Design review of the part built by this model. Coordinates are the model's own, in mm. A direction names the side the tool comes from. Coordinates: 2 decimals unless noted, no trailing zeros. Write each loop counter-clockwise with the first axis right and the second up, starting at its lowest first coordinate (ties: lowest second). Pieces come first, ordered by that corner, then holes. Notation, with made-up numbers: M -0.5,32 L 22.5,32 A13 ccw 22.5,39 Z; hole C 79.25,7 d7. An arc over 180 degrees is marked long. Return JSON: item names as keys, results as strings. Group by question number.
```python
from build123d import *

# Parameters (mm, degrees)
SKETCH1_W           = 34.124427795
SKETCH1_H           = 26.117733668
SKETCH1_R           = 1.70000044
BOSS_EXTRUDE3_DEPTH = 2.5


with BuildPart() as part:
    # Sketch1 → Boss-Extrude3 (new body)
    with BuildSketch(Plane.XY):
        with Locations((17.062213898, 13.058866834)):
            Rectangle(SKETCH1_W, SKETCH1_H)
        with Locations((17.170001507, 3.630000591)):
            Circle(SKETCH1_R, mode=Mode.SUBTRACT)
        with Locations((17.170000399, 22.630012776)):
            Circle(SKETCH1_R, mode=Mode.SUBTRACT)
        Polygon((30.684032724, 15.567255888), (28.662081374, 15.567255888), (28.662081374, 19.434703738), (5.372492357, 19.434703738), (5.372492357, 6.850018518), (28.662081374, 6.850018518), (28.662081374, 10.717466368), (30.684032724, 10.717466368), align=None, mode=Mode.SUBTRACT)
    extrude(amount=BOSS_EXTRUDE3_DEPTH)


solid = part.part
```
Item 1: Machinability: for faces 1 (the flat face through (21, 5, 0)), 2 (the flat face through (5.372, 13, 1)), which of the approach directions +Z, -Z, +X, -X, +Y, -Y give a long, thin tool a straight path to every point of the face, cutting with its end or side? Answer none if there is none.
Item 2: Add section D-D (z = 2.05). Write out the cut boundary in (x, y), plus the area to 3 significant figures.
Item 3: For line 1 (Y direction, x = 17.17, z = 1.65); line 2 (X direction, y = 3.5, z = 2); line 3 (Y direction, x = 12.5, z = 1.5), list the stretches that pass through material, from the lowest coordinate up.
Item 4: Add section B-B (y = 19). Write out the cut boundary in (x, z).
Item 5: For pin 1 (1 mm diameter, centred on x = 29.5, z = 1.5, fed in from -Y), flat-tipped, find the tip position at first contact; note if it passes through.
Item 6: The part is to be moulded in two halves that separate along Y. For faces 3 (the flat face through (17, 26.118, 1)), 4 (the cylindrical face through (18.084, 24.063, 1.232)), 5 (the flat face through (21, 5, 2.5)), say which applies: pulls with the +Y half, pulls with the -Y half, needs draft (parallel to the pull), parting line crosses it, or undercut.
Item 7: Add section C-C (x = 17.17). Write out the cut boundary in (y, z).
Item 8: Add section A-A (x = 8). Write out the cut boundary in (y, z), plus the area to 3 significant figures.
Geometry check:
{
 "1": {"face 1": "-Z, +X, -X, +Y, -Y", "face 2": "+Z, -Z"},
 "2": {"outline": "M 0,0 L 34.12,0 L 34.12,26.12 L 0,26.12 Z; hole M 5.37,6.85 L 28.66,6.85 L 28.66,10.72 L 30.68,10.72 L 30.68,15.57 L 28.66,15.57 L 28.66,19.43 L 5.37,19.43 Z; hole C 17.17,3.63 d3.4; hole C 17.17,22.63 d3.4", "area": "570 mm^2"},
 "3": {"line 1": "0 to 1.93, 5.33 to 6.85, 19.43 to 20.93, 24.33 to 26.12", "line 2": "0 to 15.47, 18.87 to 34.12", "line 3": "0 to 6.85, 19.43 to 26.12"},
 "4": {"outline": "M 0,0 L 5.37,0 L 5.37,2.5 L 0,2.5 Z; M 28.66,0 L 34.12,0 L 34.12,2.5 L 28.66,2.5 Z"},
 "5": {"pin 1": "y = 0"},
 "6": {"face 3": "pulls with the +Y half", "face 4": "undercut", "face 5": "needs draft"},
 "7": {"outline": "M 0,0 L 1.93,0 L 1.93,2.5 L 0,2.5 Z; M 5.33,0 L 6.85,0 L 6.85,2.5 L 5.33,2.5 Z; M 19.43,0 L 20.93,0 L 20.93,2.5 L 19.43,2.5 Z; M 24.33,0 L 26.12,0 L 26.12,2.5 L 24.33,2.5 Z"},
 "8": {"outline": "M 0,0 L 6.85,0 L 6.85,2.5 L 0,2.5 Z; M 19.43,0 L 26.12,0 L 26.12,2.5 L 19.43,2.5 Z", "area": "33.8 mm^2"}
}
